Model file for the job. Use its own axes, mm. Face numbers are marked on the shaded views. A direction names the side the tool comes from. Give positions to 0.01 mm unless a question says otherwise; leave off trailing zeros. Write each loop counter-clockwise with the first axis right and the second up, starting at its lowest first coordinate (ties: lowest second). Pieces come first, ordered by that corner, then holes. Notation, with made-up numbers: (84.25, 7) - (98.25, 7) arc R27 ccw to (98.25, 34) - close; hole circle Ø11 at (3.25, 38.5). An arc over 180 degrees is marked (long way). One line per item, written item: value. Start each with the question number.
(1) Cut at D-D, the plane x = -11. List the corners of the cut face in (y, z).
(2) Drop flat-ended pins along their axis: P1, Ø5, axis at y = -24.5, z = 41, coming from the -X side; P2, Ø5, axis at x = -15, y = -15, coming from the -Z side; P3, Ø1, axis at y = -28, z = 17, coming from the +X side. Give the stop position or say it passes through.
(3) Probe L1, parallel to X at y = -34.5, z = 36; L2, parallel to Z at x = -11, y = -23; L3, parallel to Z at x = -14, y = -28. List the from-to ranges inside material, lowest first.
(4) Cut at A-A, the plane x = -22.25. List the corners of the cut face in (y, z), and give its area (3 significant figures).
(5) Cut at C-C, the plane z = 21.5. List the corners of the cut face in (x, y), and give its area (3 significant figures).
(6) 3-axis set-ups, long thin cutter, end or side, ignore diameter. For the marked faces 1, 2 and 3: which of +Z, -Z, +X, -X, +Y, -Y reach the whole face in a straight line?
(7) Mould opens along Z. For the marked faces 4, 5 and 6 say: pulls with the +Z half, pulls with the -Z half, needs draft (parallel to the pull), parting line crosses it, or undercut.
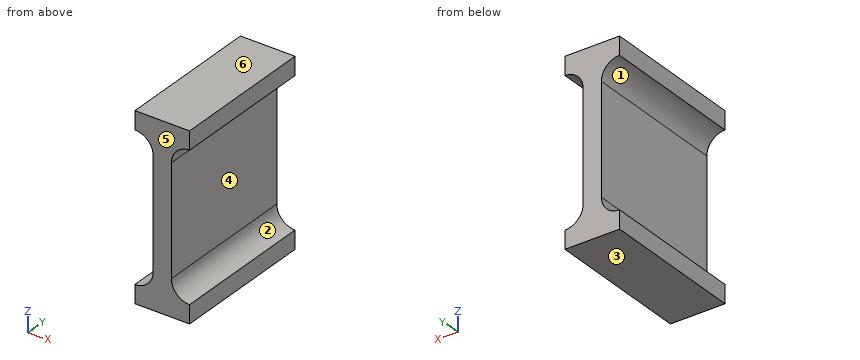
from build123d import *

# Parameters (mm, degrees)
F1_DEPTH = 40
F2_R     = 4.99999


# Not quite as in the source:
# - a fillet or chamfer is up to 0.001 mm smaller than in the source, because OpenCascade refuses the exact size


with BuildPart() as f1:
    # F0 (on Front) → F1 (new body)
    with BuildSketch(Plane.XZ):
        Polygon((-10.2562157065, 50), (-25.2562157065, 50), (-25.2562157065, 45), (-20.2562157065, 45), (-20.2562157065, 5), (-25.2562157065, 5), (-25.2562157065, 0), (-10.2562157065, 0), (-10.2562157065, 5), (-15.2562157065, 5), (-15.2562157065, 45), (-10.2562157065, 45), align=None)
    extrude(amount=F1_DEPTH)

    # F2 (radius 5 in the source; OpenCascade refuses exactly that, so slightly less here)
    f2_edges = [f1.edges().sort_by_distance(p)[0] for p in [
        (-15.256216, -20, 5),
        (-20.256216, -20, 5),
        (-15.256216, -20, 45),
        (-20.256216, -20, 45),
    ]]
    fillet(f2_edges, radius=F2_R)


solid = f1.part
Answers follow:
1. outline: (-40, 0) - (0, 0) - (0, 5.06) - (-40, 5.06) - close; (-40, 44.94) - (0, 44.94) - (0, 50) - (-40, 50) - close
2. P1: stops at x = -21.69
2. P2: stops at z = 0
2. P3: stops at x = -15.26
3. L1: x = -20.26 to -15.26
3. L2: z = 0 to 5.06, 44.94 to 50
3. L3: z = 0 to 6.69, 43.31 to 50
4. outline: (-40, 0) - (0, 0) - (0, 6) - (-40, 6) - close; (-40, 44) - (0, 44) - (0, 50) - (-40, 50) - close
4. area: 480 mm²
5. outline: (-20.26, -40) - (-15.26, -40) - (-15.26, 0) - (-20.26, 0) - close
5. area: 200 mm²
6. face 1: -X, +Y, -Y
6. face 2: +X, +Y, -Y
6. face 3: -Z, +X, -X, +Y, -Y
7. face 4: undercut
7. face 5: needs draft
7. face 6: pulls with the +Z half
